Design review of the part built by this model. Coordinates are the model's own, in mm. Coordinates: 2 decimals unless noted, no trailing zeros. Order: outer loops, then holes, each group sorted by start corner. A loop starts at its lowest first (then second) coordinate and runs counter-clockwise, first axis right, second up. Notation, with made-up numbers: (8.25, 48) -> (51.25, 48) arc R4 ccw to (51.25, 55) -> close; hole circle Ø9 at (-13.75, 45.25). An arc over 180 degrees is marked (long way). Write item = value, one per line.
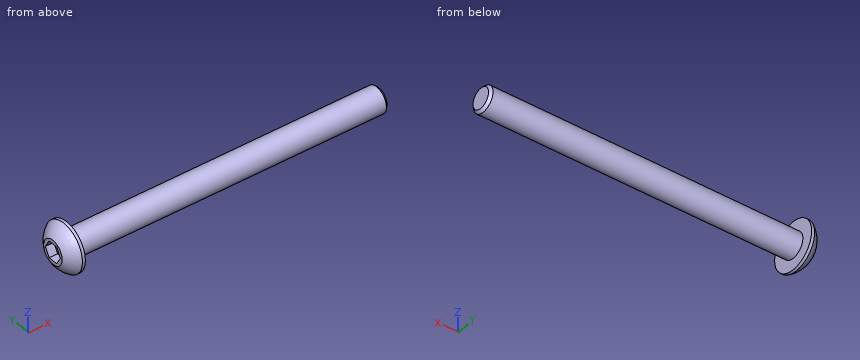
```python
from build123d import *

# Parameters (mm, degrees)
CHAMFER1_SIZE      = 0.3
CUT_EXTRUDE1_DEPTH = 1


with BuildPart() as part:
    # Sketch1 → Revolve1 (revolve)
    with BuildSketch(Plane.XY):
        with BuildLine():
            Line((38.65, 0), (0, 0))
            Line((0, 0), (0, 1.425))
            ThreePointArc((0, 1.425), (0.549895392, 2.228823502), (1.3, 2.85))
            Line((1.3, 2.85), (1.65, 2.85))
            Line((1.65, 2.85), (1.65, 1.5))
            Line((1.65, 1.5), (38.65, 1.5))
            Line((38.65, 1.5), (38.65, 0))
        make_face()
    revolve(axis=Axis((38.65, 0, 0), (-1, 0, 0)))

    # Chamfer1
    chamfer1_edges = [part.edges().sort_by_distance(p)[0] for p in [
        (38.65, -1.5, 0),
    ]]
    chamfer(chamfer1_edges, length=CHAMFER1_SIZE)

    # Sketch2 → Cut-Extrude1 (cut)
    with BuildSketch(Plane.ZY):
        Polygon((0, 1.154700538), (-1, 0.577350269), (-1, -0.577350269), (0, -1.154700538), (1, -0.577350269), (1, 0.577350269), align=None)
    extrude(amount=-CUT_EXTRUDE1_DEPTH, mode=Mode.SUBTRACT)


solid = part.part
```
(1) Insertion check: pin 1 (1 mm diameter, centred on x = 11.5, z = -1.5, fed in from +Y); pin 2 (1 mm diameter, centred on x = 27.5, z = 0, fed in from -Y); pin 3 (0.5 mm diameter, centred on x = 0.5, y = 0.5, fed in from +Z); pin 4 (1.6 mm diameter, centred on y = 0.5, z = -0.5, fed in from -X). Each pin has a flat end and moves straight along its axis. Give the tip position at first contact, or say it passes through.
Report:
pin_1 = 1.12
pin_2 = -1.5
pin_3 = 2.38
pin_4 = 0
(2) We need section A-A (x = 18). Write out the cut boundary in (y, z), and give its area (3 significant figures).
Report:
outline = circle Ø3 at (0, 0)
area = 7.07 mm²
(3) For L1, parallel to X at y = 0.45, z = 0.4; L2, parallel to Y at x = 9.5, z = -0.95; L3, parallel to X at y = 1.5, z = -2.35, list the stretches that pass through material, from the lowest coordinate up.
Report:
L1 = 1 to 38.65
L2 = -1.16 to 1.16
L3 = 1.2 to 1.65
